from build123d import *

# Parameters (mm, degrees)
SKETCH1_R               = 15.875
BOSS_EXTRUDE1_DEPTH     = 9.525
SKETCH2_R               = 9.525
SKETCH2_R_2             = 4.7625
CUT_EXTRUDE1_DEPTH      = 3.175
CUT_EXTRUDE2_DEPTH      = 25.387637749
CUT_EXTRUDE2_DEPTH_BACK = 25.387637749
SKETCH3_R               = 2.38125
FILLET2_R               = 1.5875
CHAMFER2_SIZE           = 0.396875


with BuildPart() as part:
    # Sketch1 → Boss-Extrude1 (new body)
    with BuildSketch(Plane(origin=(0, 0, 0), x_dir=(1, 0, 0), z_dir=(0, 1, 0))):
        with Locations(Location((0, 0, 0), (0, 0, 90))):
            Circle(SKETCH1_R)
    extrude(amount=BOSS_EXTRUDE1_DEPTH)

    # Sketch2 → Cut-Extrude1 (cut)
    with BuildSketch(Plane(origin=(0, 9.525, 0), x_dir=(1, 0, 0), z_dir=(0, 1, 0))):
        with Locations(Location((0, 0, 0), (0, 0, 270))):
            Circle(SKETCH2_R)
        with Locations(Location((0, 0, 0), (0, 0, 270))):
            Circle(SKETCH2_R_2, mode=Mode.SUBTRACT)
    extrude(amount=-CUT_EXTRUDE1_DEPTH, mode=Mode.SUBTRACT)

    # Sketch3 → Cut-Extrude2 (cut, two sides: drawn at the far end of the back side and taken through both)
    with BuildSketch(Plane(origin=(0, 9.525, 0), x_dir=(1, 0, 0), z_dir=(0, 1, 0)).offset(-CUT_EXTRUDE2_DEPTH_BACK)):
        with Locations(Location((0, 0, 0), (0, 0, 270))):
            Circle(SKETCH3_R)
    extrude(amount=CUT_EXTRUDE2_DEPTH + CUT_EXTRUDE2_DEPTH_BACK, mode=Mode.SUBTRACT)

    # Fillet2
    fillet2_edges = [part.edges().sort_by_distance(p)[0] for p in [
        (0, 0, 15.875),
        (0, 9.525, 15.875),
        (0, 9.525, -9.525),
    ]]
    fillet(fillet2_edges, radius=FILLET2_R)

    # Chamfer2
    chamfer2_edges = [part.edges().sort_by_distance(p)[0] for p in [
        (0, 9.525, -2.38125),
        (0, 0, -2.38125),
        (0, 6.35, -4.7625),
        (0, 9.525, -4.7625),
    ]]
    chamfer(chamfer2_edges, length=CHAMFER2_SIZE)


solid = part.part
Can you work these out from the model? Positions are in its coordinate system, mm. A direction names the side the tool comes from. Round coordinates to 2 decimals unless told otherwise and drop trailing zeros. Write item = value, one per line. Start each with the question number.
(1) For P1, Ø3, axis at x = -12, y = 2, coming from the -Z side; P2, Ø4, axis at y = 8, z = 2.5, coming from the +X side; P3, Ø8, axis at x = -4.5, z = 3, coming from the -Y side; P4, Ø3, axis at y = 1, z = 5.5, coming from the -X side, each with a flat end and sliding along its axis, tell me the tip position at first contact or that it passes through.
(2) For faces 1 (the face through (7, 9.525, 9)), 2 (the face through (-5.796, 7.155, -7.559)), which set-ups out of +Z, -Z, +X, -X, +Y, -Y let a thin tool reach every point of the face, with its end or its side?
(3) If I drill on probe 1 along X at (y, z) = (7.45, 0) (1 decimal); probe 2 along X at (y, z) = (2.75, 0) (3 decimals); probe 3 along X at (y, z) = (7.5, -1.5), over which ranges is the centre line in solid material (lowest first)? Write a range as [from, to].
(4) If we mould it in two halves opening along Z, with no side actions, what happens to faces 3 (the face through (3, 0, 0)), 4 (the face through (15.497, 4.718, 3.441)), 5 (the face through (-2.9, 7.95, -3.78)), 6 (the face through (-4, 6.35, 4))? For each: released by +Z, released by -Z, zero draft, split by the parting line, or undercut.
Ans:
q1.P1 = -11.91
q1.P2 = 15.87
q1.P3 = 0
q1.P4 = -15.34
q2.face_1 = +Z, -Z, +X, -X, +Y
q2.face_2 = +Y
q3.probe_1 = [-15.9, -9.5], [-4.8, -2.4], [2.4, 4.8], [9.5, 15.9]
q3.probe_2 = [-15.875, -2.381], [2.381, 15.875]
q3.probe_3 = [-15.8, -9.41], [-4.52, -1.85], [1.85, 4.52], [9.41, 15.8]
q4.face_3 = zero draft
q4.face_4 = split by the parting line
q4.face_5 = undercut
q4.face_6 = undercut
